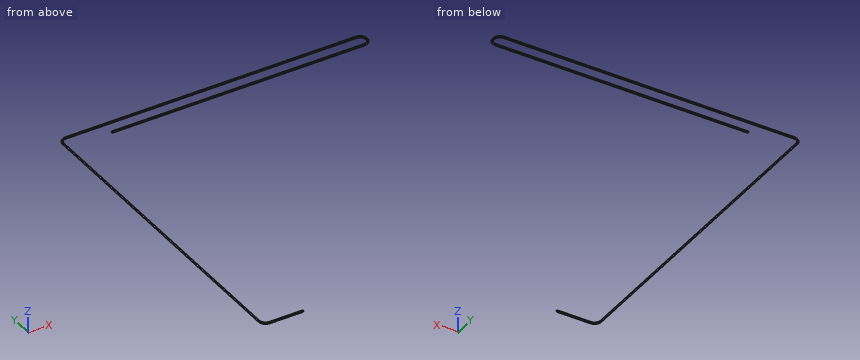
Autodesk Inventor part; units mm, degrees
ref_plane "YZ Plane" through (0, 0, 0) normal (1, 0, 0) x (0, 1, 0)
ref_plane "XZ Plane" through (0, 0, 0) normal (0, 1, 0) x (-1, 0, 0)
ref_plane "XY Plane" through (0, 0, 0) normal (0, 0, 1) x (1, 0, 0)
ref_plane "Arbeitsebene1" through (0, 0, 0) normal (0, 0, 1) x (1, 0, 0)
sketch "Skizze5" plane through (0, 0, 0) normal (0, 0, 1) x (1, 0, 0)
  circle A0 centre (0, 0) radius 10
  circle A1 centre (440, 0) radius 10
  line L0 (440, 10) -> (0, 10)
  arc A2 (0, 10) -> (-10, 0) centre (0, 0) ccw
  arc A3 (440, -10) -> (440, 10) centre (440, 0) ccw
  line L1 (440, -10) -> (57.3732, -10)
  circle A4 centre (0, -480) radius 10
  line L2 (-10, 0) -> (-10, -480)
  line L3 (0, -490) -> (50.9075, -490)
  arc A5 (-10, -480) -> (0, -490) centre (0, -480) ccw
  arc A6 (440, -10) -> (440, 10) centre (440, 0) ccw
  point P0 (0, 0)
ref_plane "Arbeitsebene4" through (57.3732, -10, 0) normal (-1, 0, 0) x (0, -1, 0)
sketch "Skizze6" plane through (57.3732, -10, 0) normal (-1, 0, 0) x (0, -1, 0)
  circle A0 centre (0, 0) radius 1
  point P0 (-10, 0)
  dimension "d3" = 2
sweep "Sweeping2" add profiles "Skizze6" path "Skizze5" path curves L1 A6 L0 A2 L2 A5 L3
properties part number "Seil1"
Work out the finished part from the listing and answer in its coordinate system (mm). Give positions to 0.01 mm unless a question says otherwise; leave off trailing zeros. Loops run counter-clockwise (first coordinate to the right, second up) from the corner with the lowest first, then second, coordinate; pieces in that order, holes last. Notation, with made-up numbers: (-5, 32) - (31, 32) arc R28 cw to (31, 66) - close; hole circle Ø9 at (-22, 77). An arc over 180 degrees is marked (long way). Answer in a Markdown table with one row per item.
(1) Consider L1, parallel to Y at x = 29.5, z = 0.05; L2, parallel to Y at x = 325, z = -0.3; L3, parallel to X at y = -366.5, z = -0.05. Determine where each line is inside the solid, lowest interval first. Write a range as [from, to].
Results list:
| item | result |
|---|---|
| L1 | y = [-491, -489], [9, 11] |
| L2 | y = [-10.95, -9.05], [9.05, 10.95] |
| L3 | x = [-11, -9] |
(2) Flat-ended cylindrical pins translate along their axes: pin 1 Ø0.6 at (y, z) = (-490, -0.5) entering from +X; pin 2 Ø0.6 at (y, z) = (-10, 0.5) entering from -X. Find the tip coordinate at first contact, or state that the pin passes through.
Results list:
| item | result |
|---|---|
| pin 1 | stops at x = 50.91 |
| pin 2 | stops at x = -10.98 |
(3) Section A-A (x = 77) is taken. Give the vertices of the cut face in (y, z).
Results list:
| item | result |
|---|---|
| outline | circle Ø2 at (-10, 0); circle Ø2 at (10, 0) |
(4) Section B-B (z = 0.4) is taken. Give the vertices of the cut face in (x, y).
Results list:
| item | result |
|---|---|
| outline | (-10.92, -480) arc R10.92 ccw to (0, -490.92) - (50.91, -490.92) - (50.91, -489.08) - (0, -489.08) arc R9.08 cw to (-9.08, -480) - (-9.08, 0) arc R9.08 cw to (0, 9.08) - (440, 9.08) arc R9.08 cw to (440, -9.08) - (57.37, -9.08) - (57.37, -10.92) - (440, -10.92) arc R10.92 ccw to (440, 10.92) - (0, 10.92) arc R10.92 ccw to (-10.92, 0) - close |
(5) Section C-C (y = -235.5) is taken. Give the vertices of the cut face in (x, z), and give its area (3 significant figures).
Results list:
| item | result |
|---|---|
| outline | circle Ø2 at (-10, 0) |
| area | 3.14 mm² |
